Model file for the job. Use its own axes, mm. Face numbers are marked on the shaded views. A direction names the side the tool comes from. Coordinates: 2 decimals unless noted, no trailing zeros. Write each loop counter-clockwise with the first axis right and the second up, starting at its lowest first coordinate (ties: lowest second). Pieces come first, ordered by that corner, then holes.
Q1. Pin check, flat tips, straight feed: P1, Ø1, axis at x = 3, y = -2.5, coming from the -Z side; P2, Ø0.7, axis at x = 1.5, z = 3.5, coming from the +Y side; P3, Ø0.8, axis at x = 0.5, z = 3.5, coming from the +Y side. Stop position of each tip, or through.
Q2. Band-saw the part on A-A, the plane x = 2.2. Write the cut outline in (y, z), plus the area to 3 significant figures.
Q3. Drill centre lines: probe 1 along Y at (x, z) = (1.65, 1.3); probe 2 along Y at (x, z) = (2.3, 2.9); probe 3 along X at (y, z) = (3.5, 2.95). Where is each one in solid material? Low to high.
Q4. Band-saw the part on D-D, the plane x = 3. Write the cut outline in (y, z), plus the area to 3 significant figures.
Q5. Band-saw the part on C-C, the plane y = 0. Write the cut outline in (x, z), plus the area to 3 significant figures.
Q6. Pull direction Y, two halves, no side cores. Call the marked faces 1, 2 and 3: released by +Y, released by -Y, zero draft, split by the parting line, or undercut.
Q7. Which spindle directions (+Z, -Z, +X, -X, +Y, -Y) get a long thin tool onto all of the face, cutting with end or side? Do the marked faces 4, 5 and 6. Say none if no direction does.
Q8. Band-saw the part on B-B, the plane z = 4. Write the cut outline in (x, y).
from build123d import *

# Parameters (mm, degrees)
AUFSATZ_LINEAR_AUSTRAGEN1_DEPTH = 6


with BuildPart() as part:
    # Skizze1 → Aufsatz-Linear austragen1 (new body)
    with BuildSketch(Plane.XY):
        with BuildLine():
            Line((0.932336104, 3.1), (1.604162004, 3.1))
            ThreePointArc((1.604162004, 3.1), (4.704162004, 0), (1.604162004, -3.1))
            Line((1.604162004, -3.1), (0.932336104, -3.1))
            Line((0.932336104, -3.1), (0.932336104, -4.1))
            Line((0.932336104, -4.1), (0, -3.723445161))
            Line((0, -3.723445161), (0, -3.356483855))
            Line((0, -3.356483855), (0, -1.9))
            Line((0, -1.9), (1.604162004, -1.9))
            ThreePointArc((1.604162004, -1.9), (3.504162004, 0), (1.604162004, 1.9))
            Line((1.604162004, 1.9), (0, 1.9))
            Line((0, 1.9), (0, 3.356483855))
            Line((0, 3.356483855), (0, 3.723445161))
            Line((0, 3.723445161), (0.932336104, 4.1))
            Line((0.932336104, 4.1), (0.932336104, 3.1))
        make_face()
    extrude(amount=AUFSATZ_LINEAR_AUSTRAGEN1_DEPTH)


solid = part.part
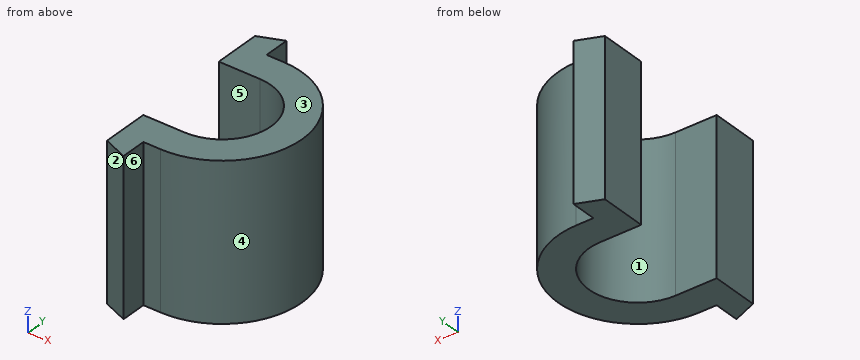
Answer sheet:
1. P1: stops at z = 0
1. P2: stops at y = 3.1
1. P3: stops at y = 4.09
2. outline: (-3.04, 0) - (-1.8, 0) - (-1.8, 6) - (-3.04, 6) - close; (1.8, 0) - (3.04, 0) - (3.04, 6) - (1.8, 6) - close
2. area: 14.9 mm2
3. probe 1: y = -3.1 to -1.9, 1.9 to 3.1
3. probe 2: y = -3.02 to -1.77, 1.77 to 3.02
3. probe 3: x = 0 to 0.93
4. outline: (-2.77, 0) - (-1.29, 0) - (-1.29, 6) - (-2.77, 6) - close; (1.29, 0) - (2.77, 0) - (2.77, 6) - (1.29, 6) - close
4. area: 17.7 mm2
5. outline: (3.5, 0) - (4.7, 0) - (4.7, 6) - (3.5, 6) - close
5. area: 7.20 mm2
6. face 1: undercut
6. face 2: released by -Y
6. face 3: zero draft
7. face 4: +Z, -Z, +X
7. face 5: +Z, -Z, -X
7. face 6: +Z, -Z, +X, -Y
8. outline: (0, -3.72) - (0.93, -4.1) - (0.93, -3.1) - (1.6, -3.1) arc R3.1 ccw to (1.6, 3.1) - (0.93, 3.1) - (0.93, 4.1) - (0, 3.72) - (0, 1.9) - (1.6, 1.9) arc R1.9 cw to (1.6, -1.9) - (0, -1.9) - close
